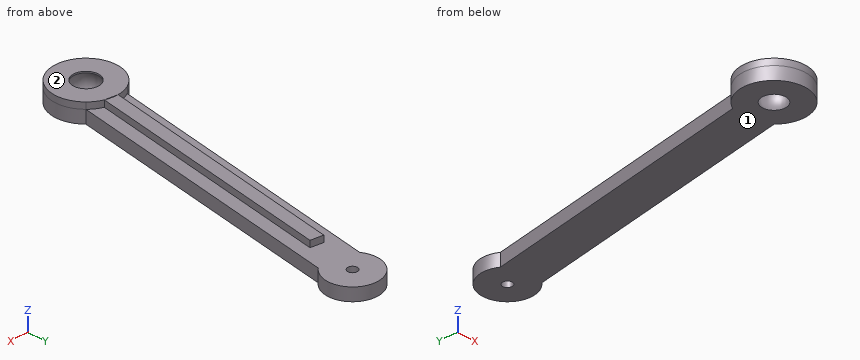
Autodesk Inventor part; units mm, degrees
ref_plane "YZ Plane" through (0, 0, 0) normal (1, 0, 0) x (0, 1, 0)
ref_plane "XZ Plane" through (0, 0, 0) normal (0, 1, 0) x (-1, 0, 0)
ref_plane "XY Plane" through (0, 0, 0) normal (0, 0, 1) x (1, 0, 0)
sketch "Sketch4" plane through (0, 0, 0) normal (0, 0, 1) x (1, 0, 0)
  circle A0 centre (0, 0) radius 0.75
  circle A1 centre (0, 0) radius 4
  spline S0 degree 3 poles (-10.1085, -50.9407) (-10.1085, -50.8779) (-10.096, -50.811) (-10.045, -50.6877) (-10.0066, -50.6315) (-9.9178, -50.5427) (-9.8616, -50.5042) (-9.7385, -50.4531) (-9.6715, -50.4405) (-9.5459, -50.4405) (-9.479, -50.453) (-9.3558, -50.5039) (-9.2995, -50.5424) (-9.2107, -50.6311) (-9.1722, -50.6873) (-9.1211, -50.8105) (-9.1085, -50.8775) (-9.1085, -51.003) (-9.121, -51.07) (-9.1719, -51.1932) (-9.2104, -51.2495) (-9.2991, -51.3383) (-9.3553, -51.3768) (-9.4785, -51.4279) (-9.5455, -51.4405) (-9.671, -51.4405) (-9.738, -51.428) (-9.8612, -51.377) (-9.9175, -51.3386) (-10.0063, -51.2498) (-10.0448, -51.1936) (-10.0959, -51.0705) (-10.1085, -51.0035) (-10.1085, -50.9407) knots 0 0 0 0 0.018836 0.018836 0.037671 0.037671 0.056507 0.056507 0.075342 0.075342 0.094178 0.094178 0.113013 0.113013 0.131849 0.131849 0.150684 0.150684 0.16952 0.16952 0.188355 0.188355 0.207191 0.207191 0.226026 0.226026 0.244862 0.244862 0.263697 0.263697 0.282533 0.282533 0.301369 0.301369 0.301369 0.301369
  spline S1 degree 3 poles (-10.1085, -50.9407) (-10.1085, -50.8779) (-10.096, -50.811) (-10.045, -50.6877) (-10.0066, -50.6315) (-9.9178, -50.5427) (-9.8616, -50.5042) (-9.7385, -50.4531) (-9.6715, -50.4405) (-9.5459, -50.4405) (-9.479, -50.453) (-9.3558, -50.5039) (-9.2995, -50.5424) (-9.2107, -50.6311) (-9.1722, -50.6873) (-9.1211, -50.8105) (-9.1085, -50.8775) (-9.1085, -51.003) (-9.121, -51.07) (-9.1719, -51.1932) (-9.2104, -51.2495) (-9.2991, -51.3383) (-9.3553, -51.3768) (-9.4785, -51.4279) (-9.5455, -51.4405) (-9.671, -51.4405) (-9.738, -51.428) (-9.8612, -51.377) (-9.9175, -51.3386) (-10.0063, -51.2498) (-10.0448, -51.1936) (-10.0959, -51.0705) (-10.1085, -51.0035) (-10.1085, -50.9407) knots 0 0 0 0 0.018836 0.018836 0.037671 0.037671 0.056507 0.056507 0.075342 0.075342 0.094178 0.094178 0.113013 0.113013 0.131849 0.131849 0.150684 0.150684 0.16952 0.16952 0.188355 0.188355 0.207191 0.207191 0.226026 0.226026 0.244862 0.244862 0.263697 0.263697 0.282533 0.282533 0.301369 0.301369 0.301369 0.301369
  circle A2 centre (-9.6085, -50.9405) radius 2.375
  circle A3 centre (-9.6085, -50.9405) radius 5
  line L0 (-9.6085, -50.9405) -> (0, 0)
  line L1 (-3.4384, -2.0438) -> (-11.8151, -46.4537)
  line L2 (-5.9191, -47.5659) -> (2.4576, -3.156)
  circle A4 centre (-9.6085, -50.9405) radius 1
  point P0 (-10.1085, -50.9407)
  dimension "d15" = 1.5
  dimension "d16" = 8
  dimension "d20" = 10
  dimension "d21" = 3
  dimension "d22" = 3
  dimension "d24" = 2
extrude "Extrusion3" add sketch "Sketch4" along normal blind 2 contours A1 | A1 L2 A3 L0 | L0 A3 L1 A1 | A3 | A2
ref_plane "Work Plane3" through (0, 0, 0) normal (0.9827, -0.1854, 0) x (0, 0, 1)
sketch "Sketch7" plane through (0, 0, 2) normal (0, 0, 1) x (1, 0, 0)
  arc A0 (-11.8151, -46.4537) -> (-5.9191, -47.5659) centre (-9.6085, -50.9405) ccw
  circle A1 centre (-9.6085, -50.9405) radius 1
  circle A2 centre (-9.6085, -50.9405) radius 5
  circle A3 centre (-9.6085, -50.9405) radius 2
  line L0 (-9.6831, -45.941) -> (-7.7178, -46.3117)
  line L1 (-7.7178, -46.3117) -> (-0.3036, -7.0049)
  line L2 (-0.3036, -7.0049) -> (-2.269, -6.6342)
  line L3 (-2.269, -6.6342) -> (-9.6831, -45.941)
  line L4 (-3.4384, -2.0438) -> (-11.8151, -46.4537)
  point P0 (0, 0)
  dimension "d26" = 4
  dimension "d27" = 2
  dimension "d28" = 40
extrude "Extrusion4" add sketch "Sketch7" along normal blind 1 contours A2 L0 A0 | L3 L2 L1 A2
sketch "Sketch8" plane through (0, 0, 0) normal (0.9827, -0.1854, 0) x (0, 0, 1)
  line L0 (2, 52.8387) -> (2, 50.8387)
  line L1 (0, 50.8387) -> (0, 52.8387)
  line L2 (3, 53.8387) -> (3, 49.8387)
  line L3 (2, 49.8387) -> (2, 53.8387)
  line L4 (0, 51.8387) -> (3, 51.8387)
  line L5 (3, 46.9398) -> (3, 46.8387)
  line L6 (0, 51.8387) -> (-0.875, 51.8387)
  line L7 (0, 47.8387) -> (0, 56.8387)
  line L8 (3, 51.8387) -> (3.875, 51.8387)
  arc A0 (3, 53.6801) -> (0, 53.6801) centre (1.5, 51.8387) ccw
  arc A1 (-0.875, 51.8387) -> (3.875, 51.8387) centre (1.5, 51.8387) ccw
  line L9 (-1.825, 51.8387) -> (4.825, 51.8387)
  point P0 (0, 0)
revolve "Revolution2" cut sketch "Sketch8" angle 360 about axis through (-9.6085, -50.9405, 0) along (0, 0, 1) contours L7 A1 L6 L1 | L1 L4 L2 A1 L7 | L2 L8 A1
equation "\"d22\" = d21"
properties part number "BackArm"
Geometry: final body of the model. Coordinates: model frame, mm. Face numbers are marked on the shaded views. Round coordinates to 2 decimals unless told otherwise and drop trailing zeros. Loops run counter-clockwise (first coordinate to the right, second up) from the corner with the lowest first, then second, coordinate; pieces in that order, holes last.
Q1. Material intervals for L1, parallel to Z at x = -5.25, y = -36; L2, parallel to X at y = -49.5, z = 0.95; L3, parallel to X at y = -52.5, z = 2.8, sorted ascending.
Q2. Section B-B on y = -44. Return loops of the section in (x, z).
Q3. Section C-C on z = 1. State how many separate pieces and enclosed holes the cut face has, plus the area to 3 significant figures.
Q4. Section A-A on y = 0. Return loops of the section in (x, z).
Q5. Pull-direction query (Z, two-part tool) for the marked faces 1 and 2; classes: released by +Z, released by -Z, zero draft, split by the parting line, or undercut.
Q6. Pin query (flat end, axial travel): P1, Ø8, axis at x = -11.5, y = -24, coming from the +Z side. Return the tip coordinate at first contact, or that it passes through.
Evaluation:
1. L1: z = 0 to 2
1. L2: x = -14.4 to -11.41, -7.8 to -4.82
1. L3: x = -14.36 to -10.86, -8.36 to -4.86
2. outline: (-11.35, 0) - (-5.25, 0) - (-5.25, 2) - (-7.28, 2) - (-7.28, 3) - (-9.32, 3) - (-9.32, 2) - (-11.35, 2) - close
3. separate pieces: 1
3. enclosed holes: 2
3. area: 372 mm2
4. outline: (-4, 0) - (-0.75, 0) - (-0.75, 2) - (-4, 2) - close; (0.75, 0) - (4, 0) - (4, 2) - (0.75, 2) - close
5. face 1: released by -Z
5. face 2: released by +Z
6. P1: stops at z = 2
